Could you check a few things on this model? Use its own coordinates, in mm. A direction names the side the tool comes from. Give positions to 0.01 mm unless a question says otherwise; leave off trailing zeros. Loops run counter-clockwise (first coordinate to the right, second up) from the corner with the lowest first, then second, coordinate; pieces in that order, holes last. Notation, with made-up numbers: (0.5, 82) -> (50.5, 82) arc R14 ccw to (50.5, 105) -> close; hole circle Ø3 at (41, 89). An arc over 180 degrees is marked (long way). Write each question's results on one line, items separated by ' | '. Start each with the question number.
Q1. We'd pull the mould along X, two halves only. Please class faces 6 (the face through (-41.275, -1, 0)), 7 (the face through (-1, -1, -9.525)), 8 (the face through (60.325, -1, 50)): released by +X, released by -X, zero draft, split by the parting line, or undercut.
Q2. Which directions (+Z, -Z, +X, -X, +Y, -Y) give clear straight access to the entire face, cutting with the end or side of a thin tool? Please do faces 1 (the face through (19, -63.5, 37)), 2 (the face through (85, -1, 38.1)), 3 (the face through (69, -1, 80.975)), 4 (the face through (45.8, -0.89, 57.15)), 5 (the face through (96, -1, 66.675)).
Q3. Will these pins go through, and if not, where does the flat tip stop? P1, Ø10, axis at y = 34.5, z = 13.5, coming from the +X side (3 decimals); P2, Ø2, axis at y = 39, z = 23, coming from the -X side; P3, Ø1.6, axis at x = 58.5, y = -1.5, coming from the -Z side; P4, Ø10, axis at x = 51, z = 7.5, coming from the -Y side.
Q4. If I drill on line 1 along X through (y, z) = (-52, 39) (3 decimals); line 2 along X through (y, z) = (-8, 44.5) (3 decimals); line 3 along Z through (x, y) = (93, -17.5) (3 decimals), over which ranges is the centre line in solid material (lowest first)?
Q5. If we section it at B-B, the plane x = 86.5: List the corners of the cut face in (y, z) for me (3 decimals).
Q6. If we section it at A-A, the plane z = -3: List the corners of the cut face in (x, y) for me (3 decimals), plus the area to 3 significant figures.
from build123d import *

# Parameters (mm, degrees)
F0_W     = 20.9652720133
F0_H     = 4.7498
F1_DEPTH = 63.5


with BuildPart() as f1:
    # F0 (on Front) → F1 (new body, symmetric)
    with BuildSketch(Plane.XZ):
        with BuildLine():
            add(Edge.make_bspline(
                [(-41.275, 9.525), (-37.169303745, 25.7526282221), (0, 81.8980410695), (57.15, 80.9752)],
                knots=[0, 0, 0, 0, 121.6248811101, 121.6248811101, 121.6248811101, 121.6248811101], degree=3))
            Line((-41.275, 9.525), (22.225, 9.525))
            Line((22.225, 9.525), (22.225, 46.0502))
            ThreePointArc((22.225, 46.0502), (32.4542956671, 70.7459043329), (57.15, 80.9752))
        make_face()
        Polygon((22.225, 9.525), (-41.275, 9.525), (-41.275, -9.525), (41.275, -9.525), (41.275, 9.525), align=None)
        with BuildLine():
            Line((22.225, 46.0502), (22.225, 9.525))
            Line((22.225, 9.525), (41.275, 9.525))
            Line((41.275, 9.525), (41.275, 46.0502))
            ThreePointArc((41.275, 46.0502), (45.9246798487, 57.2755201513), (57.15, 61.9252))
            Line((57.15, 61.9252), (60.325, 61.9252))
            Line((60.325, 61.9252), (60.325, 66.675))
            Line((60.325, 66.675), (81.2902720133, 66.675))
            Line((81.2902720133, 66.675), (81.2902720133, 80.9752))
            Line((81.2902720133, 80.9752), (57.15, 80.9752))
            ThreePointArc((57.15, 80.9752), (32.4542956671, 70.7459043329), (22.225, 46.0502))
        make_face()
        with Locations((70.8076360066, 64.3001)):
            Rectangle(F0_W, F0_H)
        Polygon((111.125, 66.675), (81.2902720133, 66.675), (81.2902720133, 61.9252), (60.325, 61.9252), (60.325, 38.1), (111.125, 38.1), align=None)
    extrude(amount=F1_DEPTH, both=True)


solid = f1.part
Final values:
1) face 6: released by -X | face 7: zero draft | face 8: undercut
2) face 1: +Z, -Z, +X, -X, -Y | face 2: -Z, +X, +Y, -Y | face 3: +Z, +X, -X, +Y, -Y | face 4: -Z, +Y, -Y | face 5: +Z, +X, +Y, -Y
3) P1: stops at x = 41.275 | P2: stops at x = -35.69 | P3: stops at z = 61.93 | P4: passes through
4) line 1: x = -23.817 to 41.275, 60.325 to 111.125 | line 2: x = -19.037 to 41.275, 60.325 to 111.125 | line 3: z = 38.1 to 66.675
5) outline: (-63.5, 38.1) -> (63.5, 38.1) -> (63.5, 66.675) -> (-63.5, 66.675) -> close
6) outline: (-41.275, -63.5) -> (41.275, -63.5) -> (41.275, 63.5) -> (-41.275, 63.5) -> close | area: 10,500 mm²
